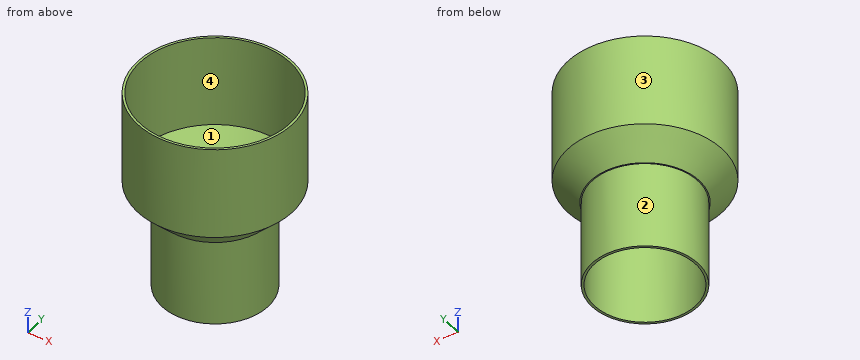
```python
from build123d import *

# Parameters (mm, degrees)
F0_R     = 11.684
F1_DEPTH = 19.05
F2_R     = 17.018
F2_R_2   = 11.684
F3_DEPTH = 25.4
F4_SIZE2 = 5.08
F4_SIZE  = 5.08
F5_T     = -0.508


with BuildPart() as f1:
    # F0 (on Top) → F1 (new body)
    with BuildSketch(Plane.XY):
        Circle(F0_R)
    extrude(amount=F1_DEPTH)

    # F2 (on face) → F3 (join)
    with BuildSketch(Plane.XY.offset(19.05)):
        Circle(F2_R)
        Circle(F2_R_2, mode=Mode.SUBTRACT)
        Circle(F2_R_2)
    extrude(amount=F3_DEPTH)

    # F4
    f4_edges = [f1.edges().sort_by_distance(p)[0] for p in [
        (-17.018, 0, 19.05),
    ]]
    chamfer(f4_edges, length=F4_SIZE, length2=F4_SIZE2)

    # F5
    f5_openings = [f1.faces().sort_by_distance(p)[0] for p in [
        (0, 0, 44.45),
        (0, 0, 0),
    ]]
    offset(amount=F5_T, openings=f5_openings, kind=Kind.INTERSECTION)


solid = f1.part
```
Geometry: final body of the model. Coordinates: model frame, mm. Face numbers are marked on the shaded views. A direction names the side the tool comes from. Give positions to 0.01 mm unless a question says otherwise; leave off trailing zeros. Loops run counter-clockwise (first coordinate to the right, second up) from the corner with the lowest first, then second, coordinate; pieces in that order, holes last. Notation, with made-up numbers: (70.25, -23) -> (94.25, -23) arc R32 ccw to (94.25, 9) -> close; hole circle Ø6 at (2, 12). An arc over 180 degrees is marked (long way). Use one line per item in the form item = value.
Item 1: Line query: probe 1 along Y at (x, z) = (0, 29); probe 2 along X at (y, z) = (3.5, 26); probe 3 along X at (y, z) = (-15, 25.5). Output: solid intervals per line, ascending.
A:
probe_1 = -17.02 to -16.51, 16.51 to 17.02
probe_2 = -16.65 to -16.13, 16.13 to 16.65
probe_3 = -8.04 to -6.9, 6.9 to 8.04
Item 2: Section query D-D on z = 25. Output: boundary loops of the cut face in (x, y), and give its area (3 significant figures).
A:
outline = circle Ø34.04 at (0, 0); hole circle Ø33.02 at (0, 0)
area = 53.5 mm^2
Item 3: Draft query along X for the marked faces 3 and 4. Return one class per face: pulls with the +X half, pulls with the -X half, needs draft (parallel to the pull), parting line crosses it, or undercut.
A:
face_3 = parting line crosses it
face_4 = undercut
Item 4: Section query C-C on z = 14.5. Output: boundary loops of the cut face in (x, y), and give its area (3 significant figures).
A:
outline = circle Ø23.37 at (0, 0); hole circle Ø22.35 at (0, 0)
area = 36.5 mm^2
Item 5: Section query A-A on x = 0. Output: boundary loops of the cut face in (y, z).
A:
outline = (-17.02, 24.13) -> (-11.94, 19.05) -> (-11.68, 19.05) -> (-11.68, 0) -> (-11.18, 0) -> (-11.18, 19.56) -> (-11.73, 19.56) -> (-16.51, 24.34) -> (-16.51, 44.45) -> (-17.02, 44.45) -> close; (11.18, 0) -> (11.68, 0) -> (11.68, 19.05) -> (11.94, 19.05) -> (17.02, 24.13) -> (17.02, 44.45) -> (16.51, 44.45) -> (16.51, 24.34) -> (11.73, 19.56) -> (11.18, 19.56) -> close
Item 6: Pin query (flat end, axial travel): P1, Ø10, axis at x = 1, z = 15, coming from the -Y side; P2, Ø4, axis at x = 10.5, y = 6, coming from the +Z side; P3, Ø2, axis at y = -9.5, z = 38.5, coming from the -X side. Return the tip coordinate at first contact, or that it passes through.
A:
P1 = -12.86
P2 = 21.92
P3 = -14.74
Item 7: Access query for the marked faces 1 and 2. Directions: +Z, -Z, +X, -X, +Y, -Y. A direction counts if a zero-diameter tool reaches every point of the face in a straight line with its end or side. Return the directions, or none.
A:
face_1 = +Z
face_2 = -Z
